```python
from build123d import *

# Parameters (mm, degrees)
SKETCH3_R           = 38.5
SKETCH3_R_2         = 32.5
BOSS_EXTRUDE3_DEPTH = 160
SKETCH5_R           = 36.7411
SKETCH5_R_2         = 35.6743
SKETCH5_R_3         = 34.6075
CUT_EXTRUDE1_DEPTH  = 1.4224
SKETCH5_4_R         = 45
SKETCH5_4_R_2       = 38.5
BOSS_EXTRUDE5_DEPTH = 5
SKETCH7_R           = 1.55
CUT_EXTRUDE2_DEPTH  = 5
CUT_EXTRUDE3_START  = -80
SKETCH9_R           = 38.5
SKETCH9_R_2         = 32.5
CUT_EXTRUDE3_DEPTH  = 80
CUT_EXTRUDE6_START  = -1.4224
SKETCH5_7_R         = 36.7411
SKETCH5_7_R_2       = 35.6743
SKETCH5_7_R_3       = 34.6075
CUT_EXTRUDE6_DEPTH  = 1.4224


with BuildPart() as part:
    # Sketch3 → Boss-Extrude3 (new body)
    with BuildSketch(Plane(origin=(0, 0, 0), x_dir=(1, 0, 0), z_dir=(0, 1, 0))):
        with Locations(Location((0, 0, 0), (0, 0, 270))):
            Circle(SKETCH3_R)
        with Locations(Location((0, 0, 0), (0, 0, 270))):
            Circle(SKETCH3_R_2, mode=Mode.SUBTRACT)
    boss_extrude3 = extrude(amount=BOSS_EXTRUDE3_DEPTH)

    # Sketch5 → Cut-Extrude1 (cut)
    # profile 1 of 2: a face of its own
    with BuildSketch(Plane.XZ):
        with Locations(Location((0, 0, 0), (0, 0, 270))):
            Circle(SKETCH5_R)
        Circle(SKETCH5_R_2, mode=Mode.SUBTRACT)
    # profile 2 of 2: a face of its own
    with BuildSketch(Plane.XZ):
        Circle(SKETCH5_R_2)
        with Locations(Location((0, 0, 0), (0, 0, 270))):
            Circle(SKETCH5_R_3, mode=Mode.SUBTRACT)
    cut_extrude1 = extrude(amount=-CUT_EXTRUDE1_DEPTH, mode=Mode.SUBTRACT)

    # Sketch5_4 → Boss-Extrude5 (add)
    with BuildSketch(Plane.XZ):
        with Locations(Location((0, 0, 0), (0, 0, 270))):
            Circle(SKETCH5_4_R)
        with Locations(Location((0, 0, 0), (0, 0, 270))):
            Circle(SKETCH5_4_R_2, mode=Mode.SUBTRACT)
    boss_extrude5 = extrude(amount=-BOSS_EXTRUDE5_DEPTH)

    # Sketch7 → Cut-Extrude2 (cut)
    with BuildSketch(Plane(origin=(0, 5, 0), x_dir=(1, 0, 0), z_dir=(0, 1, 0))):
        with Locations(Location((0, 41.75, 0), (0, 0, 270))):
            Circle(SKETCH7_R)
        with Locations(Location((29.521708115, 29.521708115, 0), (0, 0, 270))):
            Circle(SKETCH7_R)
        with Locations(Location((41.75, 0, 0), (0, 0, 270))):
            Circle(SKETCH7_R)
        with Locations(Location((29.521708115, -29.521708115, 0), (0, 0, 270))):
            Circle(SKETCH7_R)
        with Locations(Location((0, -41.75, 0), (0, 0, 270))):
            Circle(SKETCH7_R)
        with Locations(Location((-29.521708115, -29.521708115, 0), (0, 0, 270))):
            Circle(SKETCH7_R)
        with Locations(Location((-41.75, 0, 0), (0, 0, 270))):
            Circle(SKETCH7_R)
        with Locations(Location((-29.521708115, 29.521708115, 0), (0, 0, 270))):
            Circle(SKETCH7_R)
    cut_extrude2 = extrude(amount=-CUT_EXTRUDE2_DEPTH, mode=Mode.SUBTRACT)

    # Sketch9 → Cut-Extrude3 (cut)
    with BuildSketch(Plane(origin=(0, 160, 0), x_dir=(1, 0, 0), z_dir=(0, 1, 0)).offset(CUT_EXTRUDE3_START)):
        with Locations(Location((0, 0, 0), (0, 0, 90))):
            Circle(SKETCH9_R)
        with Locations(Location((0, 0, 0), (0, 0, 270))):
            Circle(SKETCH9_R_2, mode=Mode.SUBTRACT)
    extrude(amount=CUT_EXTRUDE3_DEPTH, mode=Mode.SUBTRACT)

    # Mirror7: Boss-Extrude3, Cut-Extrude1, Boss-Extrude5, Cut-Extrude2 across plane
    add(boss_extrude3.mirror(Plane.ZX.offset(80)))
    add(cut_extrude1.mirror(Plane.ZX.offset(80)), mode=Mode.SUBTRACT)
    add(boss_extrude5.mirror(Plane.ZX.offset(80)))
    add(cut_extrude2.mirror(Plane.ZX.offset(80)), mode=Mode.SUBTRACT)

    # Sketch5_7 → Cut-Extrude6 (cut)
    # profile 1 of 2: a face of its own
    with BuildSketch(Plane.XZ.offset(CUT_EXTRUDE6_START)):
        with Locations(Location((0, 0, 0), (0, 0, 270))):
            Circle(SKETCH5_7_R)
        Circle(SKETCH5_7_R_2, mode=Mode.SUBTRACT)
    # profile 2 of 2: a face of its own
    with BuildSketch(Plane.XZ.offset(CUT_EXTRUDE6_START)):
        Circle(SKETCH5_7_R_2)
        with Locations(Location((0, 0, 0), (0, 0, 270))):
            Circle(SKETCH5_7_R_3, mode=Mode.SUBTRACT)
    extrude(amount=CUT_EXTRUDE6_DEPTH, mode=Mode.SUBTRACT)


solid = part.part
```
Work out the finished part from the listing and answer in its coordinate system (mm). A direction names the side the tool comes from. Round coordinates to 2 decimals unless told otherwise and drop trailing zeros. Write each loop counter-clockwise with the first axis right and the second up, starting at its lowest first coordinate (ties: lowest second). Pieces come first, ordered by that corner, then holes. Notation, with made-up numbers: (-0.5, 24.25) - (42.5, 24.25) arc R29 ccw to (42.5, 46.25) - close; hole circle Ø5 at (60.25, 64.5). An arc over 180 degrees is marked (long way). Return JSON: item names as keys, results as strings. Group by question number.
Q1. Find the intervals of material crossed by L1, parallel to X at y = 1.25, z = 0; L2, parallel to X at y = 34, z = -0.5; L3, parallel to Y at x = 19, z = 38.5, in increasing order.
Q2. For faces 1 (the flat face through (-33, 160, 17)), 2 (the flat face through (-22, 158.578, -27)), 3 (the cylindrical face through (-33.785, 0.721, 7.502)), determine the directions among +Z, -Z, +X, -X, +Y, -Y from which every point of the face is accessible in a straight line to the end or side of a thin tool.
Q3. The mould has two halves that part along Z. Classify faces 4 (the cylindrical face through (0.466, 2.535, 43.228)), 5 (the flat face through (34, 5, -20)), 6 (the cylindrical face through (-17.235, 157.535, -41.569)): released by +Z, released by -Z, zero draft, split by the parting line, or undercut.
Q4. Each of these flat-tipped pins is pushed along its axis until it touches: pin 1 Ø4 at (x, y) = (31.5, 118) entering from +Z; pin 2 Ø4 at (x, z) = (29.52, 29.52) entering from +Y; pin 3 Ø1.5 at (x, y) = (23, 79) entering from -Z; pin 4 Ø6 at (y, z) = (51, -16) entering from -X. Where does it stop, or does it pass through?
Q5. The part is cut by section C-C on y = 135. Write down the section's boundary in (x, z), then the cut area to 3 significant figures.
Solved:
{
 "1": {"L1": "-45 to -43.3, -40.2 to -36.74, -34.61 to -32.5, 32.5 to 34.61, 36.74 to 40.2, 43.3 to 45", "L2": "-38.5 to -32.5, 32.5 to 38.5", "L3": "0 to 5, 155 to 160"},
 "2": {"face 1": "+Z, -Z, +X, -X, +Y", "face 2": "+Y", "face 3": "-Y"},
 "3": {"face 4": "undercut", "face 5": "zero draft", "face 6": "split by the parting line"},
 "4": {"pin 1": "z = 24.74", "pin 2": "y = 160", "pin 3": "z = -31.42", "pin 4": "x = -36.24"},
 "5": {"outline": "circle Ø77 at (0, 0); hole circle Ø65 at (0, 0)", "area": "1,340 mm²"}
}
